```python
from build123d import *

# Parameters (mm, degrees)
SKETCH1_R           = 12
BOSS_EXTRUDE1_DEPTH = 14
SKETCH2_R           = 10
BOSS_EXTRUDE2_DEPTH = 3
SKETCH3_R           = 8
BOSS_EXTRUDE3_DEPTH = 33
FILLET1_R           = 0.5


with BuildPart() as part:
    # Sketch1 → Boss-Extrude1 (new body)
    with BuildSketch(Plane(origin=(0, 0, 0), x_dir=(0, 0, -1), z_dir=(1, 0, 0))):
        Circle(SKETCH1_R)
    extrude(amount=BOSS_EXTRUDE1_DEPTH)

    # Sketch2 → Boss-Extrude2 (add)
    with BuildSketch(Plane(origin=(14, 0, 0), x_dir=(0, 0, -1), z_dir=(1, 0, 0))):
        Circle(SKETCH2_R)
    extrude(amount=BOSS_EXTRUDE2_DEPTH)

    # Sketch3 → Boss-Extrude3 (add)
    with BuildSketch(Plane(origin=(17, 0, 0), x_dir=(0, 0, -1), z_dir=(1, 0, 0))):
        Circle(SKETCH3_R)
    extrude(amount=BOSS_EXTRUDE3_DEPTH)

    # Fillet1
    fillet1_edges = [part.edges().sort_by_distance(p)[0] for p in [
        (17, 0, 8),
        (14, 0, 10),
    ]]
    fillet(fillet1_edges, radius=FILLET1_R)


solid = part.part
```
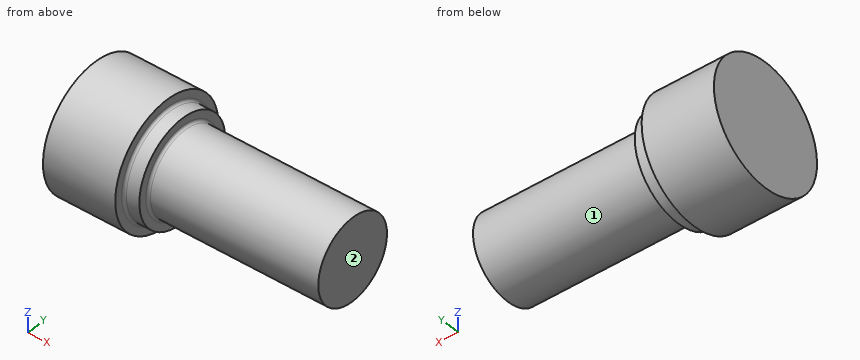
Here's how the part is built. I have some questions about the finished solid (model axes, mm). Face numbers are marked on the shaded views. A direction names the side the tool comes from. Give positions to 0.01 mm unless a question says otherwise; leave off trailing zeros. Order: outer loops, then holes, each group sorted by start corner. A loop starts at its lowest first (then second) coordinate and runs counter-clockwise, first axis right, second up. Notation, with made-up numbers: (78.25, 39) -> (125.25, 39) arc R22 cw to (125.25, 68) -> close; hole circle Ø2 at (-27.75, -12.5). An arc over 180 degrees is marked (long way). Use CSV: the item, a comma, the result in double quotes. Start each with the question number.
Item 1: If I drill on probe 1 along X at (y, z) = (-9.75, -4); probe 2 along X at (y, z) = (-9, 2.75); probe 3 along Z at (x, y) = (11, 0.25), over which ranges is the centre line in solid material (lowest first)? Write a range as [from, to].
Item 2: Suppose I cut it at C-C (x = 15.5). List the corners of the cut face in (y, z) for me, and give its area (3 significant figures).
Item 3: On a 3-axis mill with a long thin cutter (end or side, diameter ignored), from which of +Z, -Z, +X, -X, +Y, -Y can I reach the whole of each face in a straight line? I mean the marked faces 1 and 2. Say none if no direction works.
Item 4: Suppose I cut it at A-A (y = 0). List the corners of the cut face in (x, z) for me.
Item 5: Suppose I cut it at D-D (x = 23.5). List the corners of the cut face in (y, z) for me.
Item 6: I'm going to push flat-ended pins straight in: P1, Ø10, axis at x = 32.5, y = -7, coming from the -Z side; P2, Ø1.5, axis at x = 35.5, y = -7, coming from the +Z side; P3, Ø5, axis at x = 30, y = -7, coming from the +Z side. Where does each tip first touch, or does it pass through?
Answer block:
1,probe 1,"x = [0, 14]"
1,probe 2,"x = [0, 17]"
1,probe 3,"z = [-12, 12]"
2,outline,"circle Ø20 at (0, 0)"
2,area,"314 mm^2"
3,face 1,"+X"
3,face 2,"+Z, -Z, +X, +Y, -Y"
4,outline,"(0, -12) -> (14, -12) -> (14, -10.5) arc R0.5 cw to (14.5, -10) -> (17, -10) -> (17, -8.5) arc R0.5 cw to (17.5, -8) -> (50, -8) -> (50, 8) -> (17.5, 8) arc R0.5 cw to (17, 8.5) -> (17, 10) -> (14.5, 10) arc R0.5 cw to (14, 10.5) -> (14, 12) -> (0, 12) -> close"
5,outline,"circle Ø16 at (0, 0)"
6,P1,"stops at z = -7.75"
6,P2,"stops at z = 4.99"
6,P3,"stops at z = 6.61"
